Design review of the part built by this model. Coordinates are the model's own, in mm. A direction names the side the tool comes from. Coordinates: 2 decimals unless noted, no trailing zeros. Loops run counter-clockwise (first coordinate to the right, second up) from the corner with the lowest first, then second, coordinate; pieces in that order, holes last. Notation, with made-up numbers: (-26, 81) -> (24, 81) arc R9 cw to (24, 91) -> close; hole circle Ø11 at (89.25, -36.5). An arc over 180 degrees is marked (long way). Use one line per item in the form item = value. Start each with the question number.
1. Machinability: for faces 4 (the face through (0.22, 58.64, 2.1)), 5 (the face through (17.01, 16.12, 19.5)), 6 (the face through (0, -59.5, 14)), which of the approach directions +Z, -Z, +X, -X, +Y, -Y give a long, thin tool a straight path to every point of the face, cutting with its end or side? Answer none if there is none.
2. The part is to be moulded in two halves that separate along Z. For faces 1 (the face through (-17, -24, 29)), 2 (the face through (-16.99, 16.12, 19.5)), 3 (the face through (18, -1, 14)), say which applies: released by +Z, released by -Z, zero draft, split by the parting line, or undercut.
3. For pin 1 (12 mm diameter, centred on x = 0, y = 29.5, fed in from +Z); pin 2 (5 mm diameter, centred on y = -5.25, z = 14.5, fed in from -X); pin 3 (5 mm diameter, centred on x = -8, z = 7, fed in from +Y); pin 4 (1.6 mm diameter, centred on x = -17.5, z = 15, fed in from +Y), all flat-tipped, find the tip position at first contact; note any pin that passes through.
4. Consider section C-C (y = 51). State the section outline as (x, z) points.
5. Consider section A-A (y = -13.25). State the section outline as (x, z) points, then the cut area to 3 significant figures.
6. Consider section D-D (z = 6.5). State how many separate pieces and enclosed holes the cut face has, then the cut area to 3 significant figures.
7. Wall thickness on line 1 (X direction, y = 11, z = 20.25); line 2 (Z direction, x = -9, y = 19); line 3 (Y direction, x = 4.5, z = 25.75): over which ranges is each line inside the solid? List them lowest first. Write a range as from..to.
from build123d import *

# Parameters (mm, degrees)
F0_W      = 36
F0_H      = 119
F1_DEPTH  = 3
F3_DEPTH  = 26
F5_SIZE   = 25
F6_R      = 10
F7_R      = 2.99999
F8_R      = 5
F10_DEPTH = 25
F9_R      = 1.4
F9_R_2    = 4
F11_DEPTH = 36.001


# Not quite as in the source:
# - a fillet or chamfer is up to 0.001 mm smaller than in the source, because OpenCascade refuses the exact size


with BuildPart() as f1:
    # F0 (on Top) → F1 (new body)
    with BuildSketch(Plane.XY):
        Rectangle(F0_W, F0_H)
    extrude(amount=F1_DEPTH)

    # F2 (on face) → F3 (join)
    with BuildSketch(Plane.XY.offset(3)):
        Polygon((16, -57.5), (-16, -57.5), (-16, 57.5), (-16, 59.5), (-18, 59.5), (-18, -59.5), (18, -59.5), (18, 59.5), (16, 59.5), (16, 57.5), align=None)
    extrude(amount=F3_DEPTH)

    # F5
    f5_edges = [f1.edges().sort_by_distance(p)[0] for p in [
        (-17, 59.5, 29),
        (17, 59.5, 29),
    ]]
    chamfer(f5_edges, length=F5_SIZE)

    # F6
    f6_edges = [f1.edges().sort_by_distance(p)[0] for p in [
        (17, 34.5, 29),
        (-17, 34.5, 29),
    ]]
    fillet(f6_edges, radius=F6_R)

    # F7 (radius 3 in the source; OpenCascade refuses exactly that, so slightly less here)
    f7_edges = [f1.edges().sort_by_distance(p)[0] for p in [
        (0, 59.5, 3),
    ]]
    fillet(f7_edges, radius=F7_R)

    # F8
    f8_edges = [f1.edges().sort_by_distance(p)[0] for p in [
        (17, 59.5, 4),
        (-17, 59.5, 4),
    ]]
    fillet(f8_edges, radius=F8_R)

    # F4 (on face) → F10 (cut)
    with BuildSketch(Plane.XY.offset(3)):
        with BuildLine():
            ThreePointArc((-1.2459935794, 48.5), (-1.95, 47), (-1.2459935794, 45.5))
            ThreePointArc((-1.2459935794, 45.5), (0, 45.05), (1.2459935794, 45.5))
            ThreePointArc((1.2459935794, 45.5), (1.7652460848, 46.1715036149), (1.95, 47))
            ThreePointArc((1.95, 47), (1.7652460848, 47.8284963851), (1.2459935794, 48.5))
            ThreePointArc((1.2459935794, 48.5), (0, 48.95), (-1.2459935794, 48.5))
        make_face()
    extrude(amount=-F10_DEPTH, mode=Mode.SUBTRACT)

    # F9 (on face) → F11 (cut, through all)
    with BuildSketch(Plane.YZ.offset(18)):
        with Locations((-5.25, 22.5)):
            Circle(F9_R)
        with Locations((2.75, 14.5)):
            Circle(F9_R)
        with Locations((-5.25, 14.5)):
            Circle(F9_R_2)
        with Locations((-5.25, 6.5)):
            Circle(F9_R)
        with Locations((-13.25, 14.5)):
            Circle(F9_R)
        Polygon((-45.6205420196, 14.5), (-53.8677945733, 24.8276256025), (-53.8677945733, 4.6137683094), align=None)
        Polygon((-30.4197221994, 24.8276256025), (-38.6669747531, 14.5), (-30.4197221994, 4.6137683094), align=None)
        Polygon((11.8845089816, 4.5387393932), (20.1667771096, 14.395655056), (11.9562095653, 24.7524695214), align=None)
        Polygon((35.4041344278, 24.6692968517), (27.1203006313, 14.3709900539), (35.3324338441, 4.4555667236), align=None)
    extrude(amount=-F11_DEPTH, mode=Mode.SUBTRACT)


solid = f1.part
Geometry check:
q1.face_4 = +Z, +Y
q1.face_5 = +X, -X
q1.face_6 = +Z, -Z, +X, -X, -Y
q2.face_1 = released by +Z
q2.face_2 = undercut
q2.face_3 = zero draft
q3.pin_1 = 3
q3.pin_2 = through
q3.pin_3 = -57.5
q3.pin_4 = 49.3
q4.outline = (-18, 0) -> (18, 0) -> (18, 12.5) -> (16, 12.5) -> (16, 3) -> (-16, 3) -> (-16, 12.5) -> (-18, 12.5) -> close
q5.outline = (-18, 0) -> (18, 0) -> (18, 13.1) -> (16, 13.1) -> (16, 3) -> (-16, 3) -> (-16, 13.1) -> (-18, 13.1) -> close; (-18, 15.9) -> (-16, 15.9) -> (-16, 29) -> (-18, 29) -> close; (16, 15.9) -> (18, 15.9) -> (18, 29) -> (16, 29) -> close
q5.area = 201 mm²
q6.separate_pieces = 11
q6.enclosed_holes = 0
q6.area = 493 mm²
q7.line_1 = -18..-16, 16..18
q7.line_2 = 0..3
q7.line_3 = -59.5..-57.5
